Here's how the part is built. I have some questions about the finished solid (model axes, mm). Face numbers are marked on the shaded views. A direction names the side the tool comes from. Coordinates: 2 decimals unless noted, no trailing zeros. Write each loop counter-clockwise with the first axis right and the second up, starting at its lowest first coordinate (ties: lowest second). Pieces come first, ordered by that corner, then holes. Notation, with made-up numbers: (-23.75, -36) -> (-5.75, -36) arc R17 cw to (-5.75, -30) -> close; hole circle Ø4 at (60, 57.25). An arc over 180 degrees is marked (long way). Use a Markdown table: item, result. Add a question column.
Item 1: Will these pins go through, and if not, where does the flat tip stop? pin 1 Ø2 at (y, z) = (2.5, -5) entering from -X; pin 2 Ø1.3 at (x, y) = (5, 0.5) entering from -Z; pin 3 Ø6 at (x, z) = (-4.5, -8) entering from +Y; pin 4 Ø0.6 at (x, y) = (-11, 1) entering from +Z.
Item 2: On a 3-axis mill with a long thin cutter (end or side, diameter ignored), from which of +Z, -Z, +X, -X, +Y, -Y can I reach the whole of each face in a straight line? I mean the marked faces 1, 2 and 3. Say none if no direction works.
Item 3: Imagine slicing it at D-D, the plane y = 2. Write out the boundary of the cut face in (x, z).
Item 4: Imagine slicing it at A-A, the plane z = 2.5. Write out the boundary of the cut face in (x, y), and give its area (3 significant figures).
Item 5: Imagine slicing it at C-C, the plane x = -11.25. Write out the boundary of the cut face in (y, z), and give its area (3 significant figures).
Item 6: If I drill on line 1 along Y through (x, z) = (-5.75, -7.25); line 2 along Z through (x, y) = (-1.25, 1.5); line 3 along Z through (x, y) = (3.75, 0.45), over which ranges is the centre line in solid material (lowest first)? Write a range as from..to.
Item 7: Imagine slicing it at B-B, the plane y = 0.45. Write out the boundary of the cut face in (x, z).
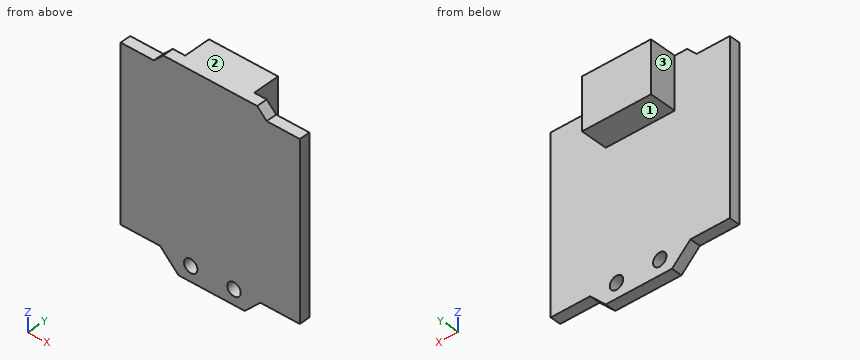
```python
from build123d import *

# Parameters (mm, degrees)
BOSS_EXTRUDE1_DEPTH = 1.2
SKETCH2_W           = 7.7
SKETCH2_H           = 5.8
BOSS_EXTRUDE2_DEPTH = 3
SKETCH5_R           = 0.75
CUT_EXTRUDE1_DEPTH  = 3


with BuildPart() as part:
    # Sketch1 → Boss-Extrude1 (new body)
    with BuildSketch(Plane(origin=(0, 0, 0), x_dir=(1, 0, 0), z_dir=(0, 1, 0))):
        Polygon((-13.031308411, -6.656542056), (-13.031308411, 12.537383178), (-8.631308411, 12.537383178), (-6.575233645, 14.593457944), (0.818691589, 14.593457944), (2.568691589, 12.843457944), (6.968691589, 12.843457944), (6.968691589, -6.656542056), (3.268691589, -6.656542056), (2.208031417, -7.717202228), (-8.270648239, -7.717202228), (-9.331308411, -6.656542056), align=None)
    extrude(amount=BOSS_EXTRUDE1_DEPTH)

    # Sketch2 → Boss-Extrude2 (add)
    with BuildSketch(Plane(origin=(0, 1.2, 0), x_dir=(1, 0, 0), z_dir=(0, 1, 0))):
        with Locations((-3.031308411, -4.817202228)):
            Rectangle(SKETCH2_W, SKETCH2_H)
    extrude(amount=BOSS_EXTRUDE2_DEPTH)

    # Sketch5 → Cut-Extrude1 (cut)
    with BuildSketch(Plane(origin=(0, 1.2, 0), x_dir=(1, 0, 0), z_dir=(0, 1, 0))):
        with Locations((-5.209653936, 12.920685244)):
            Circle(SKETCH5_R)
        with Locations((-0.377462837, 12.920685244)):
            Circle(SKETCH5_R)
    extrude(amount=-CUT_EXTRUDE1_DEPTH, mode=Mode.SUBTRACT)


solid = part.part
```
Ans:
| question | item | result |
|---|---|---|
| 1 | pin 1 | passes through |
| 1 | pin 2 | stops at z = -12.84 |
| 1 | pin 3 | stops at y = 1.2 |
| 1 | pin 4 | stops at z = 6.66 |
| 2 | face 1 | -Z, +X, -X, +Y |
| 2 | face 2 | +Z, +X, -X, +Y, -Y |
| 2 | face 3 | +Z, -Z, -X, +Y |
| 3 | outline | (-6.88, 1.92) -> (0.82, 1.92) -> (0.82, 7.72) -> (-6.88, 7.72) -> close |
| 4 | outline | (-13.03, 0) -> (6.97, 0) -> (6.97, 1.2) -> (0.82, 1.2) -> (0.82, 4.2) -> (-6.88, 4.2) -> (-6.88, 1.2) -> (-13.03, 1.2) -> close |
| 4 | area | 47.1 mm^2 |
| 5 | outline | (0, -12.54) -> (1.2, -12.54) -> (1.2, 6.66) -> (0, 6.66) -> close |
| 5 | area | 23.0 mm^2 |
| 6 | line 1 | y = 0..1.2 |
| 6 | line 2 | z = 1.92..7.72 |
| 6 | line 3 | z = -12.84..6.66 |
| 7 | outline | (-13.03, -12.54) -> (-8.63, -12.54) -> (-6.58, -14.59) -> (0.82, -14.59) -> (2.57, -12.84) -> (6.97, -12.84) -> (6.97, 6.66) -> (3.27, 6.66) -> (2.21, 7.72) -> (-8.27, 7.72) -> (-9.33, 6.66) -> (-13.03, 6.66) -> close; hole circle Ø1.5 at (-5.21, -12.92); hole circle Ø1.5 at (-0.38, -12.92) |
